from build123d import *

# Parameters (mm, degrees)
F1_DEPTH = 56
F3_D     = 15
F3_DEPTH = 20
F3_TIP   = 4.5064546427


with BuildPart() as f1:
    # F0 (on Right) → F1 (new body)
    with BuildSketch(Plane.YZ):
        Polygon((-15, 0), (0, 0), (15, 0), (15, 10), (30, 10), (30, 40), (0, 40), (-30, 40), (-30, 10), (-15, 10), align=None)
    extrude(amount=F1_DEPTH)

    # F3
    with Locations(Plane.YZ.offset(56)):
        with Locations((0, 20)):
            Hole(F3_D / 2, depth=F3_DEPTH)
            with Locations((0, 0, -(F3_DEPTH + F3_TIP / 2))):  # 118° drill point
                Cone(0, F3_D / 2, F3_TIP, mode=Mode.SUBTRACT)


solid = f1.part
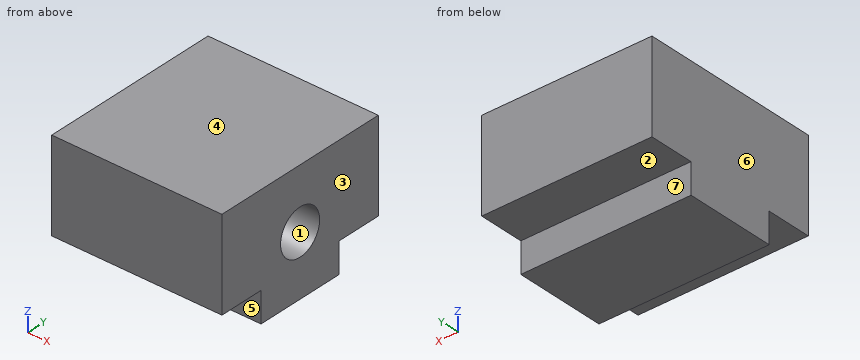
For this review, take the finished solid that the model builds, in its own axes (mm). Face numbers are marked on the shaded views. A direction names the side the tool comes from. Give positions to 0.01 mm unless a question says otherwise; leave off trailing zeros. Order: outer loops, then holes, each group sorted by start corner. A loop starts at its lowest first (then second) coordinate and runs counter-clockwise, first axis right, second up. Notation, with made-up numbers: M 21,22.5 L 53,22.5 A29 cw 53,59.5 Z; hole C 45,-15.75 d9. An arc over 180 degrees is marked long. Answer in a Markdown table with one row per item. Add a question column.
(1) Wall thickness on probe 1 along Y at (x, z) = (50.5, 20); probe 2 along Z at (x, y) = (42.75, 0); probe 3 along Z at (x, y) = (6, 18.5): over which ranges is each line inside the solid? List them lowest first. Write a range as [from, to].
(2) Consider section B-B on x = 22. State the section outline as (y, z) points.
(3) For pin 1 (10 mm diameter, centred on x = 20.5, y = -18, fed in from -Z); pin 2 (13.5 mm diameter, centred on y = 0, z = 20, fed in from +X); pin 3 (7.5 mm diameter, centred on x = 41.5, y = 22, fed in from -Z); pin 4 (5 mm diameter, centred on x = 25, z = 7, fed in from -Y), all flat-tipped, find the tip position at first contact; note any pin that passes through.
(4) Consider section D-D on y = -24. State the section outline as (x, z) points.
(5) Mouldability with a two-part tool opening along Z and no side actions: class the marked faces 1, 2, 3 and 4 as +Z half, -Z half, draft (parallel to the pull), parting line (faces both ways), or undercut.
(6) For the marked faces 5, 6 and 7, list the 3-axis set-ups (+Z, -Z, +X, -X, +Y, -Y) from which the entire face can be reached by the end or side of a thin tool; tool diameter is ignored.
(7) Consider section C-C on z = 4. State the section outline as (x, y) points.
(8) Consider section A-A on x = 52. State the section outline as (y, z) points, and give its area (3 significant figures).
Evaluation:
| question | item | result |
|---|---|---|
| 1 | probe 1 | y = [-30, -7.5], [7.5, 30] |
| 1 | probe 2 | z = [0, 12.5], [27.5, 40] |
| 1 | probe 3 | z = [10, 40] |
| 2 | outline | M -30,10 L -15,10 L -15,0 L 15,0 L 15,10 L 30,10 L 30,40 L -30,40 Z |
| 3 | pin 1 | stops at z = 0 |
| 3 | pin 2 | stops at x = 35.55 |
| 3 | pin 3 | stops at z = 10 |
| 3 | pin 4 | stops at y = -15 |
| 4 | outline | M 0,10 L 56,10 L 56,40 L 0,40 Z |
| 5 | face 1 | undercut |
| 5 | face 2 | -Z half |
| 5 | face 3 | draft |
| 5 | face 4 | +Z half |
| 6 | face 5 | -Z, +X, -X, -Y |
| 6 | face 6 | +Z, -Z, -X, +Y, -Y |
| 6 | face 7 | -Z, +X, -X, +Y |
| 7 | outline | M 0,-15 L 56,-15 L 56,15 L 0,15 Z |
| 8 | outline | M -30,10 L -15,10 L -15,0 L 15,0 L 15,10 L 30,10 L 30,40 L -30,40 Z; hole C 0,20 d15 |
| 8 | area | 1,920 mm^2 |
